Here's how the part is built. I have some questions about the finished solid (model axes, mm). Face numbers are marked on the shaded views. A direction names the side the tool comes from. Coordinates: 2 decimals unless noted, no trailing zeros. Write each loop counter-clockwise with the first axis right and the second up, starting at its lowest first coordinate (ties: lowest second). Pieces come first, ordered by that corner, then holes.
Item 1: If we mould it in two halves opening along Y, with no side actions, what happens to the marked faces 1, 2 and 3? For each: pulls with the +Y half, pulls with the -Y half, needs draft (parallel to the pull), parting line crosses it, or undercut.
Item 2: Please list where these lines run through material, in increasing order: line 1 (Y direction, x = -1.5, z = 13); line 2 (Z direction, x = -4, y = 18.5) (3 decimals); line 3 (Z direction, x = -9.5, y = 86.5).
Item 3: I want a section at A-A (z = 4.5). Please give me the cut outline in (x, y), and give its area (3 significant figures).
Item 4: I want a section at C-C (y = 34). Please give me the cut outline in (x, z) (3 decimals).
Item 5: I want a section at D-D (z = 8). Please give me the cut outline in (x, y).
Item 6: For the marked faces 4 and 5, which set-ups out of +Z, -Z, +X, -X, +Y, -Y let a thin tool reach every point of the face, with its end or its side?
Item 7: I want a section at B-B (x = -6.5). Please give me the cut outline in (y, z) (3 decimals).
Item 8: I'm going to push flat-ended pins straight in: P1, Ø5, axis at x = -26.5, y = 61.5, coming from the +Z side; P2, Ø4, axis at x = -15, y = 66, coming from the +Z side; P3, Ø6, axis at x = -15.5, y = 80, coming from the +Z side. Where does each tip first touch, or does it pass through?
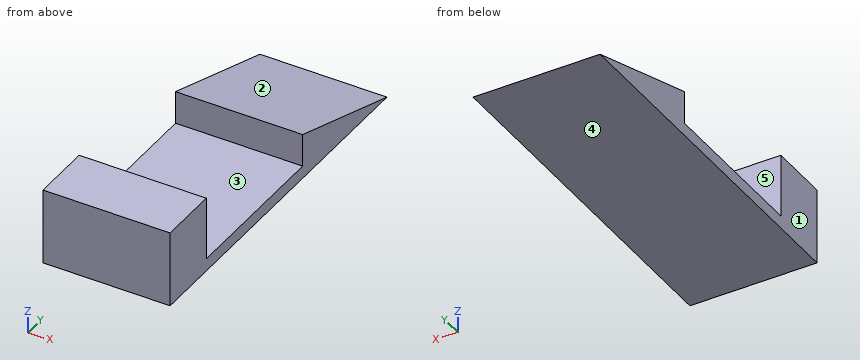
from build123d import *

# Parameters (mm, degrees)
F0_W     = 31.75
F0_H     = 40.64
F1_DEPTH = 3.175
F0_H_2   = 15.24
F2_DEPTH = 19.05
F0_H_3   = 35.56
F3_DEPTH = 11.43
F5_DEPTH = 31.75


with BuildPart() as f1:
    # F0 (on Top) → F1 (new body)
    with BuildSketch(Plane.XY):
        with Locations((-15.875, 35.56)):
            Rectangle(F0_W, F0_H)
    extrude(amount=F1_DEPTH)

    # F0 (on Top) → F2 (join)
    with BuildSketch(Plane.XY):
        with Locations((-15.875, 7.62)):
            Rectangle(F0_W, F0_H_2)
    extrude(amount=F2_DEPTH)

    # F0 (on Top) → F3 (join)
    with BuildSketch(Plane.XY):
        with Locations((-15.875, 73.66)):
            Rectangle(F0_W, F0_H_3)
    extrude(amount=F3_DEPTH)

    # F4 (on face) → F5 (cut, through all)
    with BuildSketch(Plane.YZ):
        Polygon((91.44, 11.43), (55.88, 11.43), (91.44, 0), align=None)
    extrude(amount=-F5_DEPTH, mode=Mode.SUBTRACT)


solid = f1.part
Answer:
1. face 1: needs draft
1. face 2: pulls with the +Y half
1. face 3: undercut
2. line 1: y = 0 to 15.24
2. line 2: z = 0 to 3.175
2. line 3: z = 0 to 1.59
3. outline: (-31.75, 0) - (0, 0) - (0, 15.24) - (-31.75, 15.24) - close; (-31.75, 55.88) - (0, 55.88) - (0, 77.44) - (-31.75, 77.44) - close
3. area: 1,170 mm2
4. outline: (-31.75, 0) - (0, 0) - (0, 3.175) - (-31.75, 3.175) - close
5. outline: (-31.75, 0) - (0, 0) - (0, 15.24) - (-31.75, 15.24) - close; (-31.75, 55.88) - (0, 55.88) - (0, 66.55) - (-31.75, 66.55) - close
6. face 4: -Z, +X, -X, +Y, -Y
6. face 5: +Z, +X, -X
7. outline: (0, 0) - (91.44, 0) - (55.88, 11.43) - (55.88, 3.175) - (15.24, 3.175) - (15.24, 19.05) - (0, 19.05) - close
8. P1: stops at z = 10.43
8. P2: stops at z = 8.82
8. P3: stops at z = 4.64
